Check sheet for the modelled part. Datum: model origin and axes. Units: mm. Face numbers are marked on the shaded views. A direction names the side the tool comes from. Give positions to 0.01 mm unless a question says otherwise; leave off trailing zeros. Write each loop counter-clockwise with the first axis right and the second up, starting at its lowest first coordinate (ties: lowest second). Pieces come first, ordered by that corner, then holes. Notation, with made-up numbers: M 57,36.25 L 116,36.25 A11 cw 116,55.25 Z; hole C 7.5,-26 d9. An arc over 180 degrees is marked long. Write item = value, one per line. Start each with the question number.
1) Sectioned sample at C-C, the plane z = 12.5. Record the cut outline in (x, y).
2) Sectioned sample at A-A, the plane z = -22.1. Record the cut outline in (x, y).
3) Gauge pin test, flat ends, axial feed: pin 1 (1.9 mm diameter, centred on y = -1.5, z = 9.5, fed in from -X); pin 2 (8 mm diameter, centred on x = -38, z = 4, fed in from -Y); pin 3 (3 mm diameter, centred on x = -36.13, z = 22.1, fed in from -Y); pin 4 (1 mm diameter, centred on y = -1, z = -18, fed in from +X). Record the tip position at first contact, or that the pin passes through.
4) Sectioned sample at D-D, the plane y = -2.6. Record the cut outline in (x, z).
5) Set-up check for the marked faces 1, 2 and 3: record each of +Z, -Z, +X, -X, +Y, -Y from which the full face is reachable in a straight line by a thin tool's end or side.
6) Sectioned sample at B-B, the plane x = -36.13. Record the cut outline in (y, z).
7) Scan lines: L1, parallel to Z at x = 40.05, y = 1.05; L2, parallel to X at y = -1.1, z = -21; L3, parallel to Y at x = 36.5, z = 17.5. Record each from-to range of solid material in increasing order.
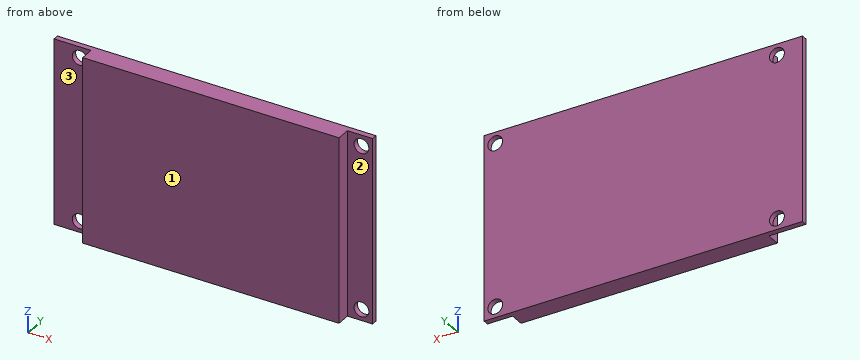
from build123d import *

# Parameters (mm, degrees)
F0_W     = 86.1
F0_H     = 50.2
F1_DEPTH = 1.5
F2_W     = 69.3
F2_H     = 50.2
F3_DEPTH = 3.75
F4_R     = 2
F5_DEPTH = 1.501


with BuildPart() as f1:
    # F0 (on Front) → F1 (new body)
    with BuildSketch(Plane.XZ):
        Rectangle(F0_W, F0_H)
    extrude(amount=-F1_DEPTH)

    # F2 (on Front) → F3 (join)
    with BuildSketch(Plane.XZ):
        with Locations((1.6, 0)):
            Rectangle(F2_W, F2_H)
    extrude(amount=F3_DEPTH)

    # F4 (on Front) → F5 (cut, through all)
    with BuildSketch(Plane.XZ):
        with Locations((-36.13, 22.1)):
            Circle(F4_R)
        with Locations((-36.13, -22.1)):
            Circle(F4_R)
        with Locations((40.05, 22.1)):
            Circle(F4_R)
        with Locations((40.05, -22.1)):
            Circle(F4_R)
    extrude(amount=-F5_DEPTH, mode=Mode.SUBTRACT)


solid = f1.part
Data:
q1.outline = M -43.05,0 L -33.05,0 L -33.05,-3.75 L 36.25,-3.75 L 36.25,0 L 43.05,0 L 43.05,1.5 L -43.05,1.5 Z
q2.outline = M -43.05,0 L -38.13,0 L -38.13,1.5 L -43.05,1.5 Z; M -34.13,0 L -33.05,0 L -33.05,-3.75 L 36.25,-3.75 L 36.25,0 L 38.05,0 L 38.05,1.5 L -34.13,1.5 Z; M 42.05,0 L 43.05,0 L 43.05,1.5 L 42.05,1.5 Z
q3.pin_1 = -33.05
q3.pin_2 = 0
q3.pin_3 = through
q3.pin_4 = 36.25
q4.outline = M -33.05,-25.1 L 36.25,-25.1 L 36.25,25.1 L -33.05,25.1 Z
q5.face_1 = +Z, -Z, +X, -X, -Y
q5.face_2 = +Z, -Z, +X, -Y
q5.face_3 = +Z, -Z, -X, -Y
q6.outline = M 0,-25.1 L 1.5,-25.1 L 1.5,-24.1 L 0,-24.1 Z; M 0,-20.1 L 1.5,-20.1 L 1.5,20.1 L 0,20.1 Z; M 0,24.1 L 1.5,24.1 L 1.5,25.1 L 0,25.1 Z
q7.L1 = -25.1 to -24.1, -20.1 to 20.1, 24.1 to 25.1
q7.L2 = -33.05 to 36.25
q7.L3 = 0 to 1.5
